Input: part model. Units: mm. Frame: model coordinates. A direction names the side the tool comes from. Give positions to 0.01 mm unless a question says otherwise; leave off trailing zeros. Loops run counter-clockwise (first coordinate to the right, second up) from the corner with the lowest first, then second, coordinate; pieces in that order, holes last. Notation, with made-up numbers: (-15, -34.75) - (0, -34.75) arc R18 cw to (0, 0.25) - close; hole circle Ø1 at (54.25, 81). An arc over 180 degrees is marked (long way). One line per question, with ' | ' between items. Start each with the question number.
from build123d import *

# Parameters (mm, degrees)
ESBO_O1_W                                            = 62
ESBO_O1_H                                            = 15
RESSALTO_EXTRUS_O1_DEPTH                             = 5
FURO_ROSCADO_PARA_CONDU_TE_DE_M3X0_51_D              = 3.15
FURO_ROSCADO_PARA_CONDU_TE_DE_M3X0_51_DEPTH          = 10
FURO_ROSCADO_PARA_CONDU_TE_DE_M3X0_51_TIP            = 0.946355475
FURO_ROSCADO_PARA_CONDU_TE_DE_M3X0_52_D              = 3.15
FURO_ROSCADO_PARA_CONDU_TE_DE_M3X0_52_DEPTH          = 7.5
FURO_ROSCADO_PARA_CONDU_TE_DE_M3X0_52_TIP            = 0.946355475
FURO_ROSCADO_PARA_CONDU_TE_DE_M2_2X0_451_D           = 2.3
ESBO_O12_W                                           = 50
ESBO_O12_H                                           = 3
RESSALTO_EXTRUS_O2_DEPTH                             = 5
ESCAREADO_PARA_PARAFUSO_DE_M_QUINA_COM_C_D           = 2.4
ESCAREADO_PARA_PARAFUSO_DE_M_QUINA_COM_C_CSINK_D     = 4.4
ESCAREADO_PARA_PARAFUSO_DE_M_QUINA_COM_C_CSINK_ANGLE = 90


with BuildPart() as part:
    # Esboço1 → Ressalto-extrusão1 (new body)
    with BuildSketch(Plane(origin=(0, 0, 0), x_dir=(1, 0, 0), z_dir=(0, 1, 0))):
        with Locations((31, 7.5)):
            Rectangle(ESBO_O1_W, ESBO_O1_H)
    extrude(amount=RESSALTO_EXTRUS_O1_DEPTH)

    # Furo roscado para conduíte de M3x0.51
    with Locations(Plane.ZY):
        with Locations((-12, 2.5), (-3, 2.5)):
            Hole(FURO_ROSCADO_PARA_CONDU_TE_DE_M3X0_51_D / 2, depth=FURO_ROSCADO_PARA_CONDU_TE_DE_M3X0_51_DEPTH)
            with Locations((0, 0, -(FURO_ROSCADO_PARA_CONDU_TE_DE_M3X0_51_DEPTH + FURO_ROSCADO_PARA_CONDU_TE_DE_M3X0_51_TIP / 2))):  # 118° drill point
                Cone(0, FURO_ROSCADO_PARA_CONDU_TE_DE_M3X0_51_D / 2, FURO_ROSCADO_PARA_CONDU_TE_DE_M3X0_51_TIP, mode=Mode.SUBTRACT)

    # Furo roscado para conduíte de M3x0.52
    with Locations(Plane(origin=(62, 0, 0), x_dir=(0, 0, -1), z_dir=(1, 0, 0))):
        with Locations((3, 2.5), (12, 2.5)):
            Hole(FURO_ROSCADO_PARA_CONDU_TE_DE_M3X0_52_D / 2, depth=FURO_ROSCADO_PARA_CONDU_TE_DE_M3X0_52_DEPTH)
            with Locations((0, 0, -(FURO_ROSCADO_PARA_CONDU_TE_DE_M3X0_52_DEPTH + FURO_ROSCADO_PARA_CONDU_TE_DE_M3X0_52_TIP / 2))):  # 118° drill point
                Cone(0, FURO_ROSCADO_PARA_CONDU_TE_DE_M3X0_52_D / 2, FURO_ROSCADO_PARA_CONDU_TE_DE_M3X0_52_TIP, mode=Mode.SUBTRACT)

    # Furo roscado para conduíte de M2.2x0.451 (through all)
    with Locations(Plane(origin=(0, 0, 0), x_dir=(-1, 0, 0), z_dir=(0, -1, 0))):
        with Locations((-4, 7.5), (-13, 7.5)):
            Hole(FURO_ROSCADO_PARA_CONDU_TE_DE_M2_2X0_451_D / 2)

    # Esboço12 → Ressalto-extrusão2 (add)
    with BuildSketch(Plane(origin=(0, 0, -15), x_dir=(-1, 0, 0), z_dir=(0, 0, -1))):
        with Locations((-31, 1.5)):
            Rectangle(ESBO_O12_W, ESBO_O12_H)
    extrude(amount=RESSALTO_EXTRUS_O2_DEPTH)

    # Escareado para parafuso de máquina com cabeça chata de M21 (through all)
    with Locations(Plane(origin=(0, 0, 0), x_dir=(-1, 0, 0), z_dir=(0, -1, 0))):
        with Locations((-11, 17.5), (-51, 17.5), (-31, 17.5)):
            CounterSinkHole(ESCAREADO_PARA_PARAFUSO_DE_M_QUINA_COM_C_D / 2, ESCAREADO_PARA_PARAFUSO_DE_M_QUINA_COM_C_CSINK_D / 2, counter_sink_angle=ESCAREADO_PARA_PARAFUSO_DE_M_QUINA_COM_C_CSINK_ANGLE)


solid = part.part
Q1. Section B-B, the plane x = 35.5. Output: boundary loops of the cut face in (y, z).
Q2. Access query for faces 1 (the face through (58.198, 3.564, -13.161)), 2 (the face through (31, 0, -10)), 3 (the face through (5.07, 2.973, -4.502)), 4 (the face through (6, 1, -17)), 5 (the face through (62, 2, -7)). Directions: +Z, -Z, +X, -X, +Y, -Y. A direction counts if a zero-diameter tool reaches every point of the face in a straight line with its end or side. Return the directions, or none.
Q3. Section C-C, the plane y = 1.95. Count the separate pieces of the cut face and the enclosed holes in it, plus the area to 3 significant figures.
Q4. Draft query along Y for faces 6 (the face through (10.782, 2.512, -12.273)), 7 (the face through (31, 3, -16)), 8 (the face through (0, 2, -7)). Return one class per face: +Y half, -Y half, draft (parallel to the pull), parting line (faces both ways), or undercut.
Q5. Line query: L1, parallel to Z at x = 6.25, y = 2.5 (3 decimals); L2, parallel to X at y = 1.9, z = -17.5; L3, parallel to X at y = 1.2, z = -7.5. Output: solid intervals per line, ascending. Write a range as from..to.
Q6. First-contact query: pin 1 (3 mm diameter, centred on x = 47.5, y = 2, fed in from +Z); pin 2 (4 mm diameter, centred on x = 11, z = -17.5, fed in from -Y); pin 3 (3 mm diameter, centred on x = 51, z = -17.5, fed in from +Y); pin 4 (1.9 mm diameter, centred on y = 2.5, z = -12, fed in from -X). Flat tips, straight axial feed; report the tip coordinate or a pass-through.
Q7. Section A-A, the plane x = 51. Output: boundary loops of the cut face in (y, z).
Solved:
1) outline: (0, -20) - (3, -20) - (3, -15) - (5, -15) - (5, 0) - (0, 0) - close
2) face 1: +X | face 2: +Z, -Z, +X, -X, -Y | face 3: -X | face 4: -Z, -X, +Y, -Y | face 5: +Z, -Z, +X, +Y, -Y
3) separate pieces: 1 | enclosed holes: 5 | area: 1,050 mm²
4) face 6: undercut | face 7: +Y half | face 8: draft
5) L1: z = -20..-13.575, -10.425..-4.575, -1.425..0 | L2: x = 6..9.8, 12.2..29.8, 32.2..49.8, 52.2..56 | L3: x = 0..2.85, 5.15..11.85, 14.15..62
6) pin 1: stops at z = 0 | pin 2: stops at y = 0.2 | pin 3: stops at y = 3 | pin 4: stops at x = 10.38
7) outline: (0, -20) - (3, -20) - (3, -18.7) - (1, -18.7) - (0, -19.7) - close; (0, -15.3) - (1, -16.3) - (3, -16.3) - (3, -15) - (5, -15) - (5, 0) - (0, 0) - close
